For this review, take the finished solid that the model builds, in its own axes (mm). Coordinates: 2 decimals unless noted, no trailing zeros. Loops run counter-clockwise (first coordinate to the right, second up) from the corner with the lowest first, then second, coordinate; pieces in that order, holes last. Notation, with made-up numbers: M 66,2 L 91,2 A15 cw 91,12 Z; hole C 69,7.25 d9. An arc over 180 degrees is marked long. Put each result on its own line as item: value.
```python
from build123d import *

# Parameters (mm, degrees)
BOSS_EXTRUDE1_DEPTH = 3.5
SKETCH2_W           = 20
SKETCH2_H           = 40
CUT_EXTRUDE1_DEPTH  = 10
CUT_EXTRUDE2_DEPTH  = 10
SKETCH4_W           = 20
SKETCH4_H           = 420
CUT_EXTRUDE3_DEPTH  = 4.5


with BuildPart() as part:
    # Sketch1 → Boss-Extrude1 (new body)
    with BuildSketch(Plane(origin=(0, 0, 0), x_dir=(1, 0, 0), z_dir=(0, 1, 0))):
        Polygon((-280, 270), (280, 270), (280, 250), (320, 250), (320, -250), (280, -250), (280, -270), (-280, -270), (-280, -250), (-320, -250), (-320, 250), (-280, 250), align=None)
    extrude(amount=BOSS_EXTRUDE1_DEPTH)

    # Sketch2 → Cut-Extrude1 (cut)
    with BuildSketch(Plane(origin=(0, 3.5, 0), x_dir=(1, 0, 0), z_dir=(0, 1, 0))):
        Polygon((30, -250), (30, -198), (-20, -198), (-20, -250), (-20, -270), (30, -270), align=None)
        Polygon((-20, 198), (30, 198), (30, 250), (30, 270), (-20, 270), (-20, 250), align=None)
        with Locations((310, 230)):
            Rectangle(SKETCH2_W, SKETCH2_H)
        with Locations((310, -230)):
            Rectangle(SKETCH2_W, SKETCH2_H)
    extrude(amount=-CUT_EXTRUDE1_DEPTH, mode=Mode.SUBTRACT)

    # Sketch3 → Cut-Extrude2 (cut)
    with BuildSketch(Plane(origin=(0, 3.5, 0), x_dir=(1, 0, 0), z_dir=(0, 1, 0))):
        with BuildLine():
            Line((149, 227), (149, 270))
            Line((149, 270), (161, 270))
            Line((161, 270), (161, 227))
            ThreePointArc((161, 227), (155, 221), (149, 227))
        make_face()
        with BuildLine():
            Line((161, -227), (161, -270))
            Line((161, -270), (149, -270))
            Line((149, -270), (149, -227))
            ThreePointArc((149, -227), (155, -221), (161, -227))
        make_face()
        with BuildLine():
            Line((-139, -227), (-139, -270))
            Line((-139, -270), (-151, -270))
            Line((-151, -270), (-151, -227))
            ThreePointArc((-151, -227), (-145, -221), (-139, -227))
        make_face()
        with BuildLine():
            Line((-151, 227), (-151, 270))
            Line((-151, 270), (-139, 270))
            Line((-139, 270), (-139, 227))
            ThreePointArc((-139, 227), (-145, 221), (-151, 227))
        make_face()
    extrude(amount=-CUT_EXTRUDE2_DEPTH, mode=Mode.SUBTRACT)

    # Sketch4 → Cut-Extrude3 (cut, through all)
    with BuildSketch(Plane(origin=(0, 3.5, 0), x_dir=(1, 0, 0), z_dir=(0, 1, 0))):
        with Locations((310, 0)):
            Rectangle(SKETCH4_W, SKETCH4_H)
    extrude(amount=-CUT_EXTRUDE3_DEPTH, mode=Mode.SUBTRACT)


solid = part.part
```
(1) Add section A-A (z = -207.5). Write out the cut boundary in (x, y), plus the area to 4 significant figures.
Determined:
outline: M -320,0 L -20,0 L -20,3.5 L -320,3.5 Z; M 30,0 L 300,0 L 300,3.5 L 30,3.5 Z
area: 1,995 mm^2
(2) For pin 1 (1 mm diameter, centred on y = 2.5, z = -260, fed in from +X); pin 2 (1.8 mm diameter, centred on x = -303.5, y = 1.5, fed in from +Z); pin 3 (1.5 mm diameter, centred on x = -14.5, y = 2.5, fed in from +Z), all flat-tipped, find the tip position at first contact; note any pin that passes through.
Determined:
pin 1: stops at x = 280
pin 2: stops at z = 250
pin 3: stops at z = 198
(3) Wall thickness on line 1 along X through (y, z) = (1.2, -205); line 2 along Z through (x, y) = (23, 1.6); line 3 along Z through (x, y) = (156, 1.1): over which ranges is each line inside the solid? List them lowest first. Write a range as [from, to].
Determined:
line 1: x = [-320, -20], [30, 300]
line 2: z = [-198, 198]
line 3: z = [-221.08, 221.08]
